Verification items for the finished model (mm, model axes). A direction names the side the tool comes from. Round coordinates to 2 decimals unless told otherwise and drop trailing zeros. Order: outer loops, then holes, each group sorted by start corner. A loop starts at its lowest first (then second) coordinate and runs counter-clockwise, first axis right, second up. Notation, with made-up numbers: (52.5, 61) -> (94.5, 61) arc R22 ccw to (94.5, 77) -> close; hole circle Ø4 at (40.5, 43). An arc over 180 degrees is marked (long way). Return JSON: item names as keys, results as strings. Group by question number.
Item 1: Sectioned sample at D-D on x = 115.5. Record the cut outline in (y, z) (3 decimals).
Item 2: Sectioned sample at A-A on x = 25.5. Record the cut outline in (y, z) (1 decimal).
Item 3: Draft check along Y on faces 1 (the flat face through (60.594, -15.557, 1.565)), 2 (the flat face through (190.53, -63.43, 1.57)), 3 (the flat face through (180.706, -73.343, 1.565)). Enter one of: pulls with the +Y half, pulls with the -Y half, needs draft (parallel to the pull), parting line crosses it, or undercut.
Item 4: Scan lines: probe 1 along Y at (x, z) = (0, 1.35); probe 2 along Y at (x, z) = (202, 1.65); probe 3 along Y at (x, z) = (6, 0.4). Record each from-to range of solid material in increasing order. Write a range as from..to.
Item 5: Sectioned sample at B-B on z = 1.4. Record the cut outline in (x, y).
Item 6: Sectioned sample at C-C on y = -69. Record the cut outline in (x, z) (3 decimals), plus the area to 3 significant figures.
Item 7: Access from +Z, -Z, +X, -X, +Y, -Y to the whole of each face (thin tool, end or side, straight path). Record for faces 4 (the flat face through (50.77, -25.47, 1.57)), 5 (the flat face through (179.048, -16.168, 1.565)), 6 (the flat face through (62.252, -72.732, 1.565)).
Item 8: Depth check by flat-ended pin: pin 1 Ø3.5 at (x, y) = (0, 0) entering from +Z. Enter the tip coordinate at first touch or a pass-through.
```python
from build123d import *

# Parameters (mm, degrees)
BOSS_EXTRUDE1_DEPTH = 3.175
SKETCH2_R           = 2.032
CUT_EXTRUDE1_DEPTH  = 266.354791982


with BuildPart() as part:
    # Sketch1 → Boss-Extrude1 (new body)
    with BuildSketch(Plane.XY):
        with BuildLine():
            Line((-2.195226767, -82.94152037), (102.281759292, -44.45004426))
            Line((102.281759292, -44.45004426), (-2.195231212, -5.958477994))
            ThreePointArc((-2.195231212, -5.958477994), (-5.95843062, 2.195359776), (2.195488341, 5.958383249))
            Line((2.195488341, 5.958383249), (120.650005048, -37.682803747))
            Line((120.650005048, -37.682803747), (239.104554312, 5.958294883))
            ThreePointArc((239.104554312, 5.958294883), (247.258439301, 2.195232145), (243.495226767, -5.958583713))
            Line((243.495226767, -5.958583713), (139.018245757, -44.450057963))
            Line((139.018245757, -44.450057963), (243.494958814, -82.941522012))
            ThreePointArc((243.494958814, -82.941522012), (247.258209334, -91.095221053), (239.104516708, -94.858485472))
            Line((239.104516708, -94.858485472), (120.65, -51.217298476))
            Line((120.65, -51.217298476), (2.195450736, -94.858397105))
            ThreePointArc((2.195450736, -94.858397105), (-5.958438371, -91.095338753), (-2.195226767, -82.94152037))
        make_face()
    extrude(amount=BOSS_EXTRUDE1_DEPTH)

    # Sketch2 → Cut-Extrude1 (cut, through all)
    with BuildSketch(Plane.XY.offset(3.175)):
        Circle(SKETCH2_R)
        with Locations((0, -88.9)):
            Circle(SKETCH2_R)
        with Locations((241.299727604, -88.9)):
            Circle(SKETCH2_R)
        with Locations((241.3, -0.000104083)):
            Circle(SKETCH2_R)
    extrude(amount=-CUT_EXTRUDE1_DEPTH, mode=Mode.SUBTRACT)


solid = part.part
```
Recorded:
{
 "1": {"outline": "(-53.115, 0) -> (-35.785, 0) -> (-35.785, 3.175) -> (-53.115, 3.175) -> close"},
 "2": {"outline": "(-86.3, 0) -> (-72.7, 0) -> (-72.7, 3.2) -> (-86.3, 3.2) -> close; (-16.2, 0) -> (-2.6, 0) -> (-2.6, 3.2) -> (-16.2, 3.2) -> close"},
 "3": {"face 1": "pulls with the +Y half", "face 2": "undercut", "face 3": "pulls with the -Y half"},
 "4": {"probe 1": "-95.25..-90.93, -86.87..-82.13, -6.77..-2.03, 2.03..6.35", "probe 2": "-81.19..-67.65, -21.25..-7.71", "probe 3": "-93.46..-79.92, -8.98..4.56"},
 "5": {"outline": "(-2.2, -82.94) arc R6.35 ccw to (2.2, -94.86) -> (120.65, -51.22) -> (239.1, -94.86) arc R6.35 ccw to (243.49, -82.94) -> (139.02, -44.45) -> (243.5, -5.96) arc R6.35 ccw to (239.1, 5.96) -> (120.65, -37.68) -> (2.2, 5.96) arc R6.35 ccw to (-2.2, -5.96) -> (102.28, -44.45) -> close; hole circle Ø4.06 at (0, -88.9); hole circle Ø4.06 at (0, 0); hole circle Ø4.06 at (241.3, -88.9); hole circle Ø4.06 at (241.3, 0)"},
 "6": {"outline": "(35.646, 0) -> (72.383, 0) -> (72.383, 3.175) -> (35.646, 3.175) -> close; (168.917, 0) -> (205.654, 0) -> (205.654, 3.175) -> (168.917, 3.175) -> close", "area": "233 mm²"},
 "7": {"face 4": "+Z, -Z, -X", "face 5": "+Z, -Z, +Y", "face 6": "+Z, -Z, -Y"},
 "8": {"pin 1": "through"}
}
